For this review, take the finished solid that the model builds, in its own axes (mm). A direction names the side the tool comes from. Coordinates: 2 decimals unless noted, no trailing zeros. Loops run counter-clockwise (first coordinate to the right, second up) from the corner with the lowest first, then second, coordinate; pieces in that order, holes last.
```python
from build123d import *

# Parameters (mm, degrees)
SKETCH1_W               = 203.2
SKETCH1_H               = 20.32
BOSS_EXTRUDE1_DEPTH     = 3.175
SKETCH2_W               = 6.35
SKETCH2_H               = 3.175
CUT_EXTRUDE1_DEPTH      = 103.156087557
LPATTERN1_COUNT         = 8
LPATTERN1_PITCH         = 25.4
MIRROR1_COPY_1_SKETCH_W = 6.35
MIRROR1_COPY_1_SKETCH_H = 3.175
MIRROR1_COPY_1_DEPTH    = 103.156087557
MIRROR1_COPY_2_SKETCH_W = 6.35
MIRROR1_COPY_2_SKETCH_H = 3.175
MIRROR1_COPY_2_DEPTH    = 103.156087557
MIRROR1_COPY_3_SKETCH_W = 6.35
MIRROR1_COPY_3_SKETCH_H = 3.175
MIRROR1_COPY_3_DEPTH    = 103.156087557
MIRROR1_COPY_4_SKETCH_W = 6.35
MIRROR1_COPY_4_SKETCH_H = 3.175
MIRROR1_COPY_4_DEPTH    = 103.156087557
MIRROR1_COPY_5_SKETCH_W = 6.35
MIRROR1_COPY_5_SKETCH_H = 3.175
MIRROR1_COPY_5_DEPTH    = 103.156087557
MIRROR1_COPY_6_SKETCH_W = 6.35
MIRROR1_COPY_6_SKETCH_H = 3.175
MIRROR1_COPY_6_DEPTH    = 103.156087557
MIRROR1_COPY_7_SKETCH_W = 6.35
MIRROR1_COPY_7_SKETCH_H = 3.175
MIRROR1_COPY_7_DEPTH    = 103.156087557
SKETCH3_W               = 6.35
SKETCH3_H               = 6.35
CUT_EXTRUDE2_DEPTH      = 103.156087557


with BuildPart() as part:
    # Sketch1 → Boss-Extrude1 (new body)
    with BuildSketch(Plane(origin=(0, 0, 0), x_dir=(1, 0, 0), z_dir=(0, 1, 0))):
        Rectangle(SKETCH1_W, SKETCH1_H)
    extrude(amount=BOSS_EXTRUDE1_DEPTH)

    # Sketch2 → Cut-Extrude1 (cut, through all)
    with BuildSketch(Plane(origin=(0, 3.175, 0), x_dir=(1, 0, 0), z_dir=(0, 1, 0))):
        with Locations((88.9, 8.5725)):
            Rectangle(SKETCH2_W, SKETCH2_H)
    cut_extrude1 = extrude(amount=-CUT_EXTRUDE1_DEPTH, mode=Mode.SUBTRACT)

    # LPattern1: Cut-Extrude1 ×8
    with Locations(*[(-i * LPATTERN1_PITCH, 0, 0) for i in range(1, LPATTERN1_COUNT)]):
        add(cut_extrude1, mode=Mode.SUBTRACT)

    # Mirror1: Cut-Extrude1 across plane
    add(cut_extrude1.mirror(Plane.XY), mode=Mode.SUBTRACT)

    # Mirror1 copy 1 sketch → Mirror1 copy 1 (cut, through all)
    with BuildSketch(Plane(origin=(-25.4, 3.175, 0), x_dir=(1, 0, 0), z_dir=(0, 1, 0))):
        with Locations((88.9, -8.5725)):
            Rectangle(MIRROR1_COPY_1_SKETCH_W, MIRROR1_COPY_1_SKETCH_H)
    extrude(amount=-MIRROR1_COPY_1_DEPTH, mode=Mode.SUBTRACT)

    # Mirror1 copy 2 sketch → Mirror1 copy 2 (cut, through all)
    with BuildSketch(Plane(origin=(-50.8, 3.175, 0), x_dir=(1, 0, 0), z_dir=(0, 1, 0))):
        with Locations((88.9, -8.5725)):
            Rectangle(MIRROR1_COPY_2_SKETCH_W, MIRROR1_COPY_2_SKETCH_H)
    extrude(amount=-MIRROR1_COPY_2_DEPTH, mode=Mode.SUBTRACT)

    # Mirror1 copy 3 sketch → Mirror1 copy 3 (cut, through all)
    with BuildSketch(Plane(origin=(-76.2, 3.175, 0), x_dir=(1, 0, 0), z_dir=(0, 1, 0))):
        with Locations((88.9, -8.5725)):
            Rectangle(MIRROR1_COPY_3_SKETCH_W, MIRROR1_COPY_3_SKETCH_H)
    extrude(amount=-MIRROR1_COPY_3_DEPTH, mode=Mode.SUBTRACT)

    # Mirror1 copy 4 sketch → Mirror1 copy 4 (cut, through all)
    with BuildSketch(Plane(origin=(-101.6, 3.175, 0), x_dir=(1, 0, 0), z_dir=(0, 1, 0))):
        with Locations((88.9, -8.5725)):
            Rectangle(MIRROR1_COPY_4_SKETCH_W, MIRROR1_COPY_4_SKETCH_H)
    extrude(amount=-MIRROR1_COPY_4_DEPTH, mode=Mode.SUBTRACT)

    # Mirror1 copy 5 sketch → Mirror1 copy 5 (cut, through all)
    with BuildSketch(Plane(origin=(-127, 3.175, 0), x_dir=(1, 0, 0), z_dir=(0, 1, 0))):
        with Locations((88.9, -8.5725)):
            Rectangle(MIRROR1_COPY_5_SKETCH_W, MIRROR1_COPY_5_SKETCH_H)
    extrude(amount=-MIRROR1_COPY_5_DEPTH, mode=Mode.SUBTRACT)

    # Mirror1 copy 6 sketch → Mirror1 copy 6 (cut, through all)
    with BuildSketch(Plane(origin=(-152.4, 3.175, 0), x_dir=(1, 0, 0), z_dir=(0, 1, 0))):
        with Locations((88.9, -8.5725)):
            Rectangle(MIRROR1_COPY_6_SKETCH_W, MIRROR1_COPY_6_SKETCH_H)
    extrude(amount=-MIRROR1_COPY_6_DEPTH, mode=Mode.SUBTRACT)

    # Mirror1 copy 7 sketch → Mirror1 copy 7 (cut, through all)
    with BuildSketch(Plane(origin=(-177.8, 3.175, 0), x_dir=(1, 0, 0), z_dir=(0, 1, 0))):
        with Locations((88.9, -8.5725)):
            Rectangle(MIRROR1_COPY_7_SKETCH_W, MIRROR1_COPY_7_SKETCH_H)
    extrude(amount=-MIRROR1_COPY_7_DEPTH, mode=Mode.SUBTRACT)

    # Sketch3 → Cut-Extrude2 (cut, through all)
    with BuildSketch(Plane(origin=(0, 3.175, 0), x_dir=(1, 0, 0), z_dir=(0, 1, 0))):
        with Locations((101.6, 0)):
            Rectangle(SKETCH3_W, SKETCH3_H)
        with Locations((-101.6, 0)):
            Rectangle(SKETCH3_W, SKETCH3_H)
    extrude(amount=-CUT_EXTRUDE2_DEPTH, mode=Mode.SUBTRACT)


solid = part.part
```
Q1. The part is to be moulded in two halves that separate along X. For faces 5 (the face through (-101.6, 2, 7)), 6 (the face through (9.525, 2, -9)), 7 (the face through (-1, 3.175, 0)), say which applies: +X half, -X half, draft (parallel to the pull), parting line (faces both ways), or undercut.
Q2. Wall thickness on probe 1 along Z at (x, y) = (65.5, 2.7) (3 decimals); probe 2 along X at (y, z) = (0.25, -3) (3 decimals): over which ranges is each line inside the solid? List them lowest first.
Q3. Machinability: for faces 1 (the face through (13, 2, -6.985)), 2 (the face through (-100, 2, 3.175)), 3 (the face through (100, 2, 3.175)), 4 (the face through (-89, 2, 6.985)), which of the approach directions +Z, -Z, +X, -X, +Y, -Y give a long, thin tool a straight path to every point of the face, cutting with its end or side? Answer none if there is none.
Q4. For pin 1 Ø1.6 at (x, y) = (-38, 2) entering from -Z (3 decimals), flat-tipped, find the tip position at first contact; note if it passes through.
Q5. Consider section A-A (z = 1.5). State the section outline as (x, y) points (3 decimals).
Q6. Consider section B-B (x = -62). State the section outline as (y, z) points (3 decimals), then the cut area to 3 significant figures.
Model answer:
1. face 5: -X half
1. face 6: undercut
1. face 7: draft
2. probe 1: z = -6.985 to 6.985
2. probe 2: x = -98.425 to 98.425
3. face 1: -Z, +Y, -Y
3. face 2: -X, +Y, -Y
3. face 3: +X, +Y, -Y
3. face 4: +Z, +Y, -Y
4. pin 1: stops at z = -6.985
5. outline: (-98.425, 0) - (98.425, 0) - (98.425, 3.175) - (-98.425, 3.175) - close
6. outline: (0, -6.985) - (3.175, -6.985) - (3.175, 6.985) - (0, 6.985) - close
6. area: 44.4 mm2
